Build history of the part. All positions in model axes, mm. Face numbers are marked on the shaded views. A direction names the side the tool comes from. Coordinates: 2 decimals unless noted, no trailing zeros. Write each loop counter-clockwise with the first axis right and the second up, starting at its lowest first coordinate (ties: lowest second). Pieces come first, ordered by that corner, then holes.
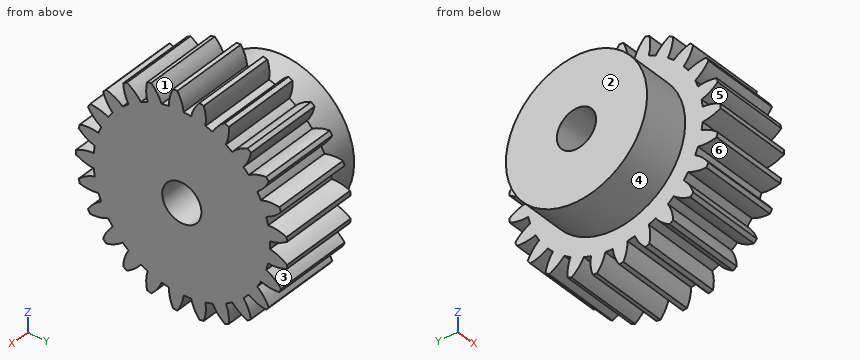
```python
from build123d import *

# Parameters (mm, degrees)
BASPROSKE_W      = 10
BASPROSKE_H      = 13.5
TOOTHCUT_DEPTH   = 22.552262062
TEETHCUTS_COUNT  = 25
TEETHCUTS_ANGLE  = 345.6
HUBNEAONESKE_R   = 9
HUBNEARONE_DEPTH = 6.0000508
BORSKE_R         = 2.5
BORE_DEPTH       = 16.0000508


with BuildPart() as part:
    # BasProSke → Base-Revolve (revolve)
    with BuildSketch(Plane(origin=(0, 0, 0), x_dir=(1, 0, 0), z_dir=(0, 1, 0)), mode=Mode.PRIVATE) as base_revolve_sk:
        with Locations((5, 6.75)):
            Rectangle(BASPROSKE_W, BASPROSKE_H)
    revolve(base_revolve_sk.sketch.rotate(Axis((-10, 0, 0), (1, 0, 0)), 180), axis=Axis((-10, 0, 0), (1, 0, 0)))

    # TooCutSke → ToothCut (cut, through all)
    with BuildSketch(Plane(origin=(0, 0, 0), x_dir=(0, 0, -1), z_dir=(1, 0, 0))):
        with BuildLine():
            ThreePointArc((0.480087995, 11.238750665), (0, 11.249), (-0.480087995, 11.238750665))
            ThreePointArc((-0.480087995, 11.238750665), (-0.821124963, 12.40220054), (-1.432168974, 13.449361962))
            ThreePointArc((-1.432168974, 13.449361962), (0, 13.5254), (1.432168974, 13.449361962))
            ThreePointArc((1.432168974, 13.449361962), (0.821124963, 12.40220054), (0.480087995, 11.238750665))
        make_face()
    toothcut = extrude(amount=TOOTHCUT_DEPTH, mode=Mode.SUBTRACT)

    # TeethCuts: ToothCut ×25 about axis
    teethcuts_axis = Axis((-10, 0, 0), (1, 0, 0))
    for i in range(1, TEETHCUTS_COUNT):
        add(toothcut.rotate(teethcuts_axis, i * TEETHCUTS_ANGLE / (TEETHCUTS_COUNT - 1)), mode=Mode.SUBTRACT)

    # HubNeaOneSke → HubNearOne (add)
    with BuildSketch(Plane.ZY):
        with Locations(Location((0, 0, 0), (0, 0, 180))):
            Circle(HUBNEAONESKE_R)
    extrude(amount=HUBNEARONE_DEPTH)

    # BorSke → Bore (cut, symmetric)
    with BuildSketch(Plane(origin=(0, 0, 0), x_dir=(0, 0, -1), z_dir=(1, 0, 0))):
        with Locations(Location((0, 0, 0), (0, 0, 180))):
            Circle(BORSKE_R)
    extrude(amount=BORE_DEPTH, both=True, mode=Mode.SUBTRACT)


solid = part.part
```
1. Flat gauge pins, fed straight in: pin 1 (2 mm diameter, centred on x = 3.5, z = -5, fed in from +Y); pin 2 (6 mm diameter, centred on x = 4.5, z = 2, fed in from +Y); pin 3 (2 mm diameter, centred on x = 7.5, y = -3.5, fed in from -Z). Where does each tip first touch, or does it go through?
Computed values:
pin 1: stops at y = 12.65
pin 2: stops at y = 13.43
pin 3: stops at z = -12.92
2. Saw through at A-A on x = -1.5. List the corners of the cut face in (y, z).
Computed values:
outline: circle Ø18 at (0, 0); hole circle Ø5 at (0, 0)
3. Mould opens along Z. For the marked faces 1, 2 and 3 say: +Z half, -Z half, draft (parallel to the pull), parting line (faces both ways), or undercut.
Computed values:
face 1: +Z half
face 2: draft
face 3: undercut
4. Probe line 1 along Y through (x, z) = (-2, 0); line 2 along Y through (x, z) = (5, 0); line 3 along Z through (x, y) = (1.5, -12). List the from-to ranges inside material, lowest first.
Computed values:
line 1: y = -9 to -2.5, 2.5 to 9
line 2: y = -13.5 to -2.5, 2.5 to 11.25
line 3: z = -3.79 to -2.26, -0.84 to 0.84, 2.26 to 3.79
5. Saw through at B-B on z = 4.25. List the corners of the cut face in (x, y), plus the area to 3 significant figures.
Computed values:
outline: (-6, -7.93) - (0, -7.93) - (0, -10.42) - (10, -10.42) - (10, 12.24) - (0, 12.24) - (0, 7.93) - (-6, 7.93) - close
area: 322 mm2
6. 3-axis set-ups, long thin cutter, end or side, ignore diameter. For the marked faces 4, 5 and 6: which of +Z, -Z, +X, -X, +Y, -Y reach the whole face in a straight line?
Computed values:
face 4: -X
face 5: +X, -X, -Y
face 6: +X, -X
